```python
from build123d import *

# Parameters (mm, degrees)
SKETCH1_W           = 148
SKETCH1_H           = 40
BOSS_EXTRUDE1_DEPTH = 30
CUT_EXTRUDE1_DEPTH  = 30
CUT_EXTRUDE2_DEPTH  = 28
FILLET1_R           = 1.6


with BuildPart() as part:
    # Sketch1 → Boss-Extrude1 (new body)
    with BuildSketch(Plane.XY):
        Rectangle(SKETCH1_W, SKETCH1_H)
    extrude(amount=BOSS_EXTRUDE1_DEPTH)

    # Sketch2 → Cut-Extrude1 (cut)
    with BuildSketch(Plane.XY.offset(30)):
        with BuildLine():
            Line((69.227207794, 17.772792206), (73.727238034, 22.272822446))
            Line((73.727238034, 22.272822446), (76.272822446, 19.727238034))
            Line((76.272822446, 19.727238034), (71.772792206, 15.227207794))
            ThreePointArc((71.772792206, 15.227207794), (69.227207794, 15.227207794), (69.227207794, 17.772792206))
        make_face()
        with BuildLine():
            Line((-69.227207794, -17.772792206), (-73.727238034, -22.272822446))
            Line((-73.727238034, -22.272822446), (-76.272822446, -19.727238034))
            Line((-76.272822446, -19.727238034), (-71.772792206, -15.227207794))
            ThreePointArc((-71.772792206, -15.227207794), (-69.227207794, -15.227207794), (-69.227207794, -17.772792206))
        make_face()
    extrude(amount=-CUT_EXTRUDE1_DEPTH, mode=Mode.SUBTRACT)

    # Sketch3 → Cut-Extrude2 (cut)
    with BuildSketch(Plane.XY.offset(30)):
        with BuildLine():
            Line((64, 27.706839185), (64, 16.5))
            ThreePointArc((64, 16.5), (65.903805922, 11.903805922), (70.5, 10))
            Line((70.5, 10), (82.036431888, 10))
            Line((82.036431888, 10), (64, 27.706839185))
        make_face()
        with BuildLine():
            Line((-64, -27.706839185), (-64, -16.5))
            ThreePointArc((-64, -16.5), (-65.903805922, -11.903805922), (-70.5, -10))
            Line((-70.5, -10), (-82.036431888, -10))
            Line((-82.036431888, -10), (-64, -27.706839185))
        make_face()
    extrude(amount=-CUT_EXTRUDE2_DEPTH, mode=Mode.SUBTRACT)

    # Fillet1
    fillet1_edges = [part.edges().sort_by_distance(p)[0] for p in [
        (-74, 5, 30),
        (74, -5, 30),
        (-5, 20, 30),
        (74, 10, 16),
        (64, 20, 16),
        (72.25, 10, 30),
        (64, 18.25, 30),
        (65.903805922, 11.903805922, 30),
        (-74, 20, 15),
        (5, -20, 30),
        (-74, -10, 16),
        (-64, -20, 16),
        (-72.25, -10, 30),
        (-64, -18.25, 30),
        (-65.903805922, -11.903805922, 30),
    ]]
    fillet(fillet1_edges, radius=FILLET1_R)


solid = part.part
```
Geometry: final body of the model. Coordinates: model frame, mm. A direction names the side the tool comes from. Round coordinates to 2 decimals unless told otherwise and drop trailing zeros. Order: outer loops, then holes, each group sorted by start corner. A loop starts at its lowest first (then second) coordinate and runs counter-clockwise, first axis right, second up. Notation, with made-up numbers: (-37.5, 61) -> (11.5, 61) arc R20 ccw to (11.5, 78) -> close; hole circle Ø2 at (87, 86.25). An arc over 180 degrees is marked (long way). Use one line per item in the form item = value. Start each with the question number.
1. Draft query along Y for faces 1 (the face through (-69.256, -15.2, 1.014)), 2 (the face through (-65.854, -11.955, 15.385)), 3 (the face through (-1, 0, 0)). Return one class per face: pulls with the +Y half, pulls with the -Y half, needs draft (parallel to the pull), parting line crosses it, or undercut.
2. Cut plane A-A (z = 24.75). Return the cut outline in (x, y).
3. Pin query (flat end, axial travel): pin 1 Ø8 at (x, y) = (54.5, -11.5) entering from -Z; pin 2 Ø0.6 at (y, z) = (17.5, 18) entering from +X; pin 3 Ø1.5 at (y, z) = (-17.5, 20.5) entering from -X; pin 4 Ø1 at (x, z) = (-71.5, 13) entering from -Y. Return the tip coordinate at first contact, or that it passes through.
4. Reachability of faces 4 (the face through (65.854, 11.955, 15.385)), 5 (the face through (-1, 20, 14)), 6 (the face through (-68, -14, 2)) from +Z, -Z, +X, -X, +Y, -Y: full face, straight path, thin tool, end or side. Return the list, or none.
5. Line query: probe 1 along X at (y, z) = (14, 3); probe 2 along X at (y, z) = (15, 26.5); probe 3 along Y at (x, z) = (-63, 25.75). Output: solid intervals per line, ascending.
Solution:
q1.face_1 = undercut
q1.face_2 = pulls with the -Y half
q1.face_3 = needs draft
q2.outline = (-74, -8.4) arc R1.6 ccw to (-72.4, -10) -> (-70.5, -10) arc R6.5 cw to (-64, -16.5) -> (-64, -18.4) arc R1.6 ccw to (-62.4, -20) -> (74, -20) -> (74, 8.4) arc R1.6 ccw to (72.4, 10) -> (70.5, 10) arc R6.5 cw to (64, 16.5) -> (64, 18.4) arc R1.6 ccw to (62.4, 20) -> (-72.4, 20) arc R1.6 ccw to (-74, 18.4) -> close
q3.pin_1 = 0
q3.pin_2 = 64
q3.pin_3 = -64
q3.pin_4 = -10
q4.face_4 = +Z, +X, +Y
q4.face_5 = +Z, -Z, +X, -X, +Y
q4.face_6 = +Z, -X, -Y
q5.probe_1 = -74 to 64.5
q5.probe_2 = -74 to 64.18
q5.probe_3 = -19.88 to 20
